Answer from the drawing. Dimensions are ordinates in mm from the lowest x, y and z of the part. Round coordinates to 2 decimals unless told otherwise and drop trailing zeros. Loops run counter-clockwise (first coordinate to the right, second up) from the corner with the lowest first, then second, coordinate; pieces in that order, holes last. Notation, with made-up numbers: (25, 52) - (42, 52) arc R26 cw to (42, 67) - close; hole circle Ø8 at (43, -16). An arc over 180 degrees is marked (long way). Return JSON: item names as keys, results as strings.
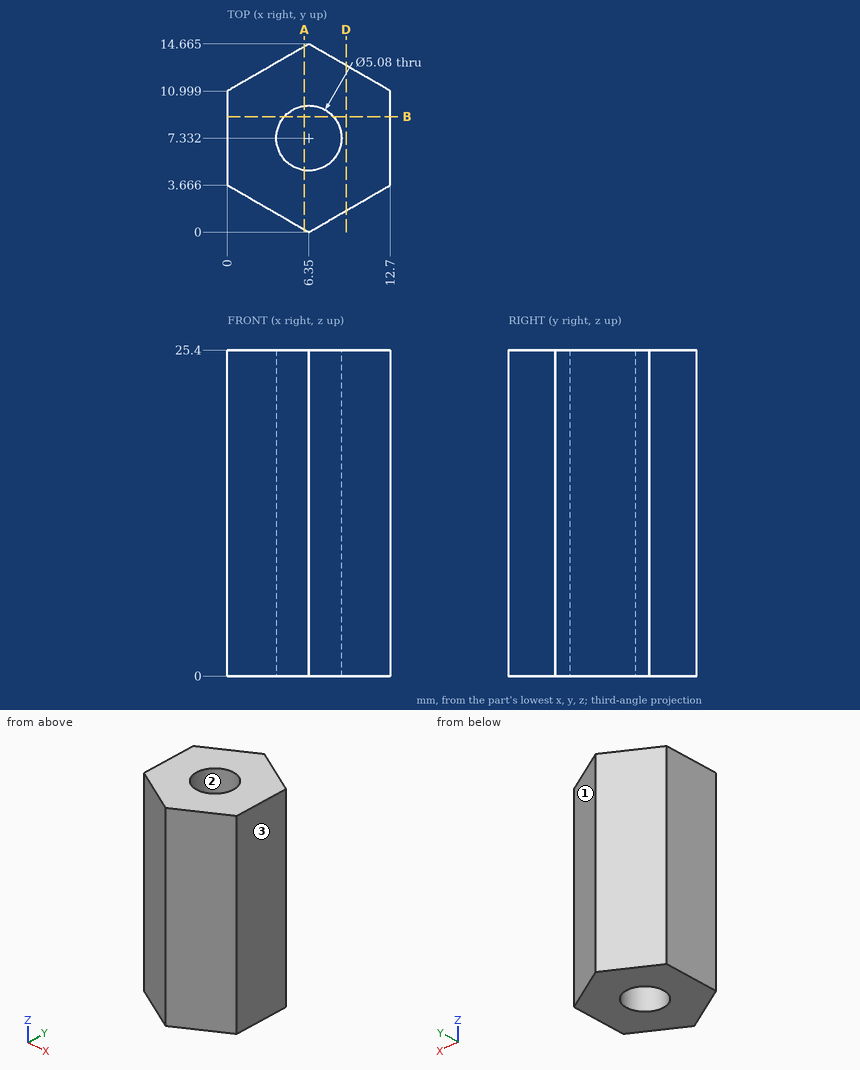
1) Flat-ended cylindrical pins translate along their axes: pin 1 (4 mm diameter, centred on x = 10.5, z = 22.5, fed in from +Y); pin 2 (6 mm diameter, centred on x = 10.5, z = 13, fed in from +Y); pin 3 (1.5 mm diameter, centred on x = 9, z = 17.5, fed in from +Y). Find the tip coordinate at first contact, or state that the pin passes through.
Verdict:
{"pin 1": "stops at y = 13.42", "pin 2": "stops at y = 14", "pin 3": "stops at y = 13.57"}
2) Section A-A (x = 6) is taken. Give the vertices of the cut face in (y, z).
Verdict:
{"outline": "(0.2, 0) - (4.82, 0) - (4.82, 25.4) - (0.2, 25.4) - close; (9.85, 0) - (14.46, 0) - (14.46, 25.4) - (9.85, 25.4) - close"}
3) Section D-D (x = 9.25) is taken. Give the vertices of the cut face in (y, z) (1 decimal).
Verdict:
{"outline": "(1.7, 0) - (13, 0) - (13, 25.4) - (1.7, 25.4) - close"}
4) Section B-B (y = 9) is taken. Give the vertices of the cut face in (x, z) (1 decimal), and give its area (3 significant figures).
Verdict:
{"outline": "(0, 0) - (4.4, 0) - (4.4, 25.4) - (0, 25.4) - close; (8.3, 0) - (12.7, 0) - (12.7, 25.4) - (8.3, 25.4) - close", "area": "225 mm2"}
5) Find the intervals of material crossed by L1, parallel to X at y = 7.25, z = 13.5; L2, parallel to X at y = 8, z = 16; L3, parallel to Y at x = 7, z = 21.5 (1 decimal), in increasing order.
Verdict:
{"L1": "x = 0 to 3.81, 8.89 to 12.7", "L2": "x = 0 to 3.9, 8.8 to 12.7", "L3": "y = 0.4 to 4.9, 9.8 to 14.3"}
6) Determine the mould class of the marked faces 1, 2 and 3 for opening direction Y: pulls with the +Y half, pulls with the -Y half, needs draft (parallel to the pull), parting line crosses it, or undercut.
Verdict:
{"face 1": "pulls with the +Y half", "face 2": "undercut", "face 3": "needs draft"}
